from build123d import *

# Parameters (mm, degrees)
BOSS_EXTRUDE1_DEPTH     = 2.5
CUT_EXTRUDE1_DEPTH      = 106.356743667
CUT_EXTRUDE1_DEPTH_BACK = 106.356743667


with BuildPart() as part:
    # Sketch1 → Boss-Extrude1 (new body)
    with BuildSketch(Plane(origin=(0, 0, 0), x_dir=(1, 0, 0), z_dir=(0, 1, 0))):
        with BuildLine():
            Line((-11.530082988, 4.75), (100.469917012, 4.75))
            ThreePointArc((100.469917012, 4.75), (105.219917012, 0), (100.469917012, -4.75))
            Line((100.469917012, -4.75), (-11.530082988, -4.75))
            ThreePointArc((-11.530082988, -4.75), (-16.280082988, 0), (-11.530082988, 4.75))
        make_face()
    extrude(amount=BOSS_EXTRUDE1_DEPTH)

    # Sketch2 → Cut-Extrude1 (cut, two sides: drawn at the far end of the back side and taken through both)
    with BuildSketch(Plane(origin=(0, 2.5, 0), x_dir=(1, 0, 0), z_dir=(0, 1, 0)).offset(-CUT_EXTRUDE1_DEPTH_BACK)):
        with BuildLine():
            Line((87.954451806, 2.025316283), (91.523765465, 2.025316283))
            ThreePointArc((91.523765465, 2.025316283), (92.364108635, 0.100316283), (91.523765465, -1.824683717))
            Line((91.523765465, -1.824683717), (87.954451806, -1.824683717))
            ThreePointArc((87.954451806, -1.824683717), (87.114108635, 0.100316283), (87.954451806, 2.025316283))
        make_face()
    extrude(amount=CUT_EXTRUDE1_DEPTH + CUT_EXTRUDE1_DEPTH_BACK, mode=Mode.SUBTRACT)


solid = part.part
Verification items for the finished model (mm, model axes). A direction names the side the tool comes from. Give positions to 0.01 mm unless a question says otherwise; leave off trailing zeros. Write each loop counter-clockwise with the first axis right and the second up, starting at its lowest first coordinate (ties: lowest second). Pieces come first, ordered by that corner, then holes. Notation, with made-up numbers: (64, 4) -> (104, 4) arc R16 ccw to (104, 16) -> close; hole circle Ø6 at (26, -12.75). An arc over 180 degrees is marked (long way). Use CSV: the item, a comma, the result in double quotes.
(1) Sectioned sample at A-A (z = 0.75). Record the cut outline in (x, y).
Derived:
outline,"(-16.22, 0) -> (87.26, 0) -> (87.26, 2.5) -> (-16.22, 2.5) -> close; (92.22, 0) -> (105.16, 0) -> (105.16, 2.5) -> (92.22, 2.5) -> close"
(2) Sectioned sample at B-B (y = 0.8). Record the cut outline in (x, z) (3 decimals).
Derived:
outline,"(-11.53, -4.75) -> (100.47, -4.75) arc R4.75 ccw to (100.47, 4.75) -> (-11.53, 4.75) arc R4.75 ccw to start; hole (87.954, -2.025) -> (91.524, -2.025) arc R2.625 ccw to (91.524, 1.825) -> (87.954, 1.825) arc R2.625 ccw to start"
(3) Set-up check for faces 1 (the cylindrical face through (87.114, 1.233, -0.07)), 2 (the cylindrical face through (105.22, 1.23, -0.1)): record each of +Z, -Z, +X, -X, +Y, -Y from which the full face is reachable in a straight line by a thin tool's end or side.
Derived:
face 1,"+Y, -Y"
face 2,"+X, +Y, -Y"
(4) Material ranges on L1, parallel to X at y = 1.55, z = 1; L2, parallel to X at y = 0.45, z = 3.5; L3, parallel to X at y = 0.9, z = 2, recorded low to high.
Derived:
L1,"x = -16.17 to 87.36, 92.12 to 105.11"
L2,"x = -14.74 to 103.68"
L3,"x = -15.84 to 104.78"
(5) Release check for a two-part mould opening along Z. For faces 3 (the flat face through (90, 1, 1.825)), 4 (the flat face through (45, 2.5, 0)), 5 (the flat face through (44, 1, -4.75)) record: +Z half, -Z half, draft (parallel to the pull), parting line (faces both ways), or undercut.
Derived:
face 3,"undercut"
face 4,"draft"
face 5,"-Z half"
